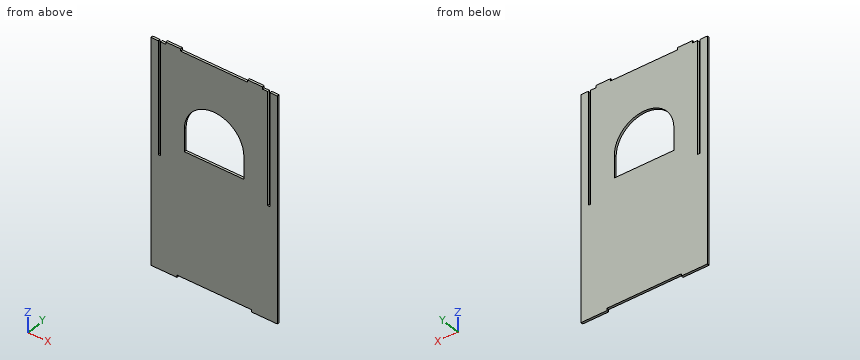
```python
from build123d import *

# Parameters (mm, degrees)
BOSS_EXTRUDE1_DEPTH = 6
SKETCH2_W           = 6
SKETCH2_H           = 300
CUT_EXTRUDE1_DEPTH  = 6
LPATTERN1_COUNT     = 2
LPATTERN1_PITCH     = 294
SKETCH3_W           = 200
SKETCH3_H           = 6
CUT_EXTRUDE2_DEPTH  = 6


with BuildPart() as part:
    # Sketch1 → Boss-Extrude1 (new body)
    with BuildSketch(Plane(origin=(0, 0, 0), x_dir=(1, 0, 0), z_dir=(0, 1, 0))):
        Polygon((300, 0), (300, -6), (260, -6), (260, 0), (80, 0), (80, -6), (40, -6), (40, 0), (0, 0), (0, 600), (340, 600), (340, 0), align=None)
    extrude(amount=BOSS_EXTRUDE1_DEPTH)

    # Sketch2 → Cut-Extrude1 (cut)
    with BuildSketch(Plane(origin=(0, 6, 0), x_dir=(1, 0, 0), z_dir=(0, 1, 0))):
        with Locations((23, 150)):
            Rectangle(SKETCH2_W, SKETCH2_H)
    cut_extrude1 = extrude(amount=-CUT_EXTRUDE1_DEPTH, mode=Mode.SUBTRACT)

    # LPattern1: Cut-Extrude1 ×2
    with Locations(*[(i * LPATTERN1_PITCH, 0, 0) for i in range(1, LPATTERN1_COUNT)]):
        add(cut_extrude1, mode=Mode.SUBTRACT)

    # Sketch3 → Cut-Extrude2 (cut)
    with BuildSketch(Plane(origin=(0, 6, 0), x_dir=(1, 0, 0), z_dir=(0, 1, 0))):
        with BuildLine():
            Line((90, 200), (90, 260))
            Line((90, 260), (250, 260))
            Line((250, 260), (250, 200))
            ThreePointArc((250, 200), (170, 120), (90, 200))
        make_face()
        with Locations((170, 597)):
            Rectangle(SKETCH3_W, SKETCH3_H)
    extrude(amount=-CUT_EXTRUDE2_DEPTH, mode=Mode.SUBTRACT)


solid = part.part
```
Design review of the part built by this model. Coordinates are the model's own, in mm. Coordinates: 2 decimals unless noted, no trailing zeros. Write each loop counter-clockwise with the first axis right and the second up, starting at its lowest first coordinate (ties: lowest second). Pieces come first, ordered by that corner, then holes. Notation, with made-up numbers: M 68.25,46 L 118.25,46 A11 cw 118.25,60 Z; hole C -19.5,26 d10. An arc over 180 degrees is marked long. Answer as a JSON object with one key per item and string values.
Item 1: Insertion check: pin 1 Ø1.8 at (x, y) = (30, 3) entering from +Z; pin 2 Ø6 at (x, z) = (101, -254.5) entering from -Y; pin 3 Ø1.8 at (y, z) = (4.5, 2) entering from +X. Each pin has a flat end and moves straight along its axis. Give the tip position at first contact, or say it passes through.
Outcome:
{"pin 1": "z = 0", "pin 2": "through", "pin 3": "x = 300"}
Item 2: Add section B-B, the plane y = 4.55. Give the boundary of the cut face in (x, z).
Outcome:
{"outline": "M 0,-600 L 70,-600 L 70,-594 L 270,-594 L 270,-600 L 340,-600 L 340,0 L 320,0 L 320,-300 L 314,-300 L 314,0 L 300,0 L 300,6 L 260,6 L 260,0 L 80,0 L 80,6 L 40,6 L 40,0 L 26,0 L 26,-300 L 20,-300 L 20,0 L 0,0 Z; hole M 90,-260 L 250,-260 L 250,-200 A80 ccw 90,-200 Z"}
Item 3: Add section A-A, the plane x = 170. Give the boundary of the cut face in (y, z), and give its area (3 significant figures).
Outcome:
{"outline": "M 0,-594 L 6,-594 L 6,-260 L 0,-260 Z; M 0,-120 L 6,-120 L 6,0 L 0,0 Z", "area": "2,720 mm²"}
Item 4: Add section C-C, the plane z = -73. Give the boundary of the cut face in (x, y), and give its area (3 significant figures).
Outcome:
{"outline": "M 0,0 L 20,0 L 20,6 L 0,6 Z; M 26,0 L 314,0 L 314,6 L 26,6 Z; M 320,0 L 340,0 L 340,6 L 320,6 Z", "area": "1,970 mm²"}
Item 5: Wall thickness on probe 1 along X at (y, z) = (2.65, -59); probe 2 along X at (y, z) = (3.45, -204.5); probe 3 along Z at (x, y) = (202.5, 0.7): over which ranges is each line inside the solid? List them lowest first.
Outcome:
{"probe 1": "0 to 20, 26 to 314, 320 to 340", "probe 2": "0 to 20, 26 to 90, 250 to 314, 320 to 340", "probe 3": "-594 to -260, -126.9 to 0"}
